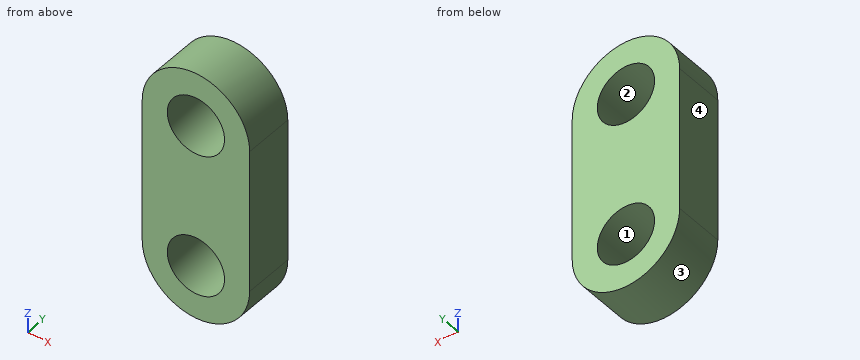
Autodesk Inventor part; units mm, degrees
ref_plane "YZ Plane" through (0, 0, 0) normal (1, 0, 0) x (0, 1, 0)
ref_plane "XZ Plane" through (0, 0, 0) normal (0, 1, 0) x (-1, 0, 0)
ref_plane "XY Plane" through (0, 0, 0) normal (0, 0, 1) x (1, 0, 0)
sketch "Sketch1" plane through (0, 0, 0) normal (0, 1, 0) x (-1, 0, 0)
  line L0 (0, 5) -> (0, -5)
  circle A0 centre (0, 5) radius 2
  circle A1 centre (0, -5) radius 2
  line L1 (0, 5) -> (0, -5) construction
  line L2 (-3.75, 5) -> (-3.75, -5)
  line L3 (3.75, -5) -> (3.75, 5)
  arc A2 (3.75, 5) -> (-3.75, 5) centre (0, 5) ccw
  arc A3 (-3.75, -5) -> (3.75, -5) centre (0, -5) ccw
  point P0 (0, 0)
  point P1 (0, 0)
  dimension "d0" = 10
  dimension "d1" = 4
  dimension "d2" = 4
  dimension "d3" = 7.5
extrude "Extrusion1" add sketch "Sketch1" along normal blind 3.5
properties part number "piulita"
Input: part model. Units: mm. Frame: model coordinates. Face numbers are marked on the shaded views. Give positions to 0.01 mm unless a question says otherwise; leave off trailing zeros. Order: outer loops, then holes, each group sorted by start corner. A loop starts at its lowest first (then second) coordinate and runs counter-clockwise, first axis right, second up. Notation, with made-up numbers: (20, 10.25) - (59, 10.25) arc R28 cw to (59, 33.25) - close; hole circle Ø9 at (76.5, 47.5). An arc over 180 degrees is marked (long way). Write each question's results on one line, items separated by ' | '.
Item 1: Material intervals for line 1 along Z through (x, y) = (0, 2.1); line 2 along X through (y, z) = (1.65, -5); line 3 along Z through (x, y) = (-1.75, 0.6), sorted ascending.
A:
line 1: z = -8.75 to -7, -3 to 3, 7 to 8.75 | line 2: x = -3.75 to -2, 2 to 3.75 | line 3: z = -8.32 to -5.97, -4.03 to 4.03, 5.97 to 8.32
Item 2: Draft query along Z for the marked faces 1, 2, 3 and 4. Return one class per face: released by +Z, released by -Z, zero draft, split by the parting line, or undercut.
A:
face 1: undercut | face 2: undercut | face 3: released by -Z | face 4: zero draft
Item 3: Contact query for flat-ended pins moving along their axis: pin 1 Ø2 at (y, z) = (0.5, 6.5) entering from -X; pin 2 Ø1 at (x, y) = (-2.5, 0.5) entering from +Z. Output: stop coordinate, or through.
A:
pin 1: stops at x = -3.72 | pin 2: stops at z = 8.17
Item 4: Section A-A (x = 0). Return loops of the section in (y, z), and give its area (4 significant figures).
A:
outline: (0, -8.75) - (3.5, -8.75) - (3.5, -7) - (0, -7) - close; (0, -3) - (3.5, -3) - (3.5, 3) - (0, 3) - close; (0, 7) - (3.5, 7) - (3.5, 8.75) - (0, 8.75) - close | area: 33.25 mm^2
Item 5: Section B-B (z = 5.75). Return loops of the section in (x, y), and give its area (3 significant figures).
A:
outline: (-3.67, 0) - (-1.85, 0) - (-1.85, 3.5) - (-3.67, 3.5) - close; (1.85, 0) - (3.67, 0) - (3.67, 3.5) - (1.85, 3.5) - close | area: 12.7 mm^2
Item 6: Section D-D (x = 2.5). Return loops of the section in (y, z).
A:
outline: (0, -7.8) - (3.5, -7.8) - (3.5, 7.8) - (0, 7.8) - close
Item 7: Section C-C (y = 2.9). Return loops of the section in (x, z).
A:
outline: (-3.75, -5) arc R3.75 ccw to (3.75, -5) - (3.75, 5) arc R3.75 ccw to (-3.75, 5) - close; hole circle Ø4 at (0, -5); hole circle Ø4 at (0, 5)
